from build123d import *

# Parameters (mm, degrees)
SKETCH1_R           = 1.79994
SKETCH1_R_2         = 1.5
BOSS_EXTRUDE1_DEPTH = 7
SKETCH2_W           = 75
SKETCH2_H           = 13.099999962
SKETCH2_R           = 2.6999438
SKETCH2_R_2         = 2.499995
SKETCH2_R_3         = 1.3498449
BOSS_EXTRUDE2_DEPTH = 6.987999994
SKETCH2_3_R         = 2.6999438
SKETCH2_3_R_2       = 1.3498449
CUT_EXTRUDE1_DEPTH  = 2.5
SKETCH7_W           = 45.754771374
SKETCH7_H           = 7.378762064
SKETCH7_W_2         = 5.75825354
SKETCH7_H_2         = 4.98011117
BOSS_EXTRUDE4_DEPTH = 7
SKETCH8_W           = 15.938133918
SKETCH8_H           = 10.613167284
CUT_EXTRUDE3_DEPTH  = 21.288
FILLET3_R           = 3.048
SKETCH4_W           = 25
SKETCH4_H           = 15.064836289
CUT_EXTRUDE2_DEPTH  = 38.822


with BuildPart() as part:
    # Sketch1 → Boss-Extrude1 (new body)
    with BuildSketch(Plane.XY):
        with BuildLine():
            Line((37.5, -10.5), (30, -10.5))
            ThreePointArc((30, -10.5), (25, -15.5), (20, -10.5))
            Line((20, -10.5), (5, -10.5))
            ThreePointArc((5, -10.5), (0, -15.5), (-5, -10.5))
            Line((-5, -10.5), (-20, -10.5))
            ThreePointArc((-20, -10.5), (-25, -15.5), (-30, -10.5))
            Line((-30, -10.5), (-37.5, -10.5))
            Line((-37.5, -10.5), (-37.5, 10.5))
            Line((-37.5, 10.5), (37.5, 10.5))
            Line((37.5, 10.5), (37.5, -10.5))
        make_face()
        with Locations((-25, -10.5)):
            Circle(SKETCH1_R, mode=Mode.SUBTRACT)
        with Locations((0, -10.5)):
            Circle(SKETCH1_R, mode=Mode.SUBTRACT)
        with Locations((25, -10.5)):
            Circle(SKETCH1_R, mode=Mode.SUBTRACT)
        with Locations((-35, 8)):
            Circle(SKETCH1_R_2, mode=Mode.SUBTRACT)
        with Locations((-15, 8)):
            Circle(SKETCH1_R_2, mode=Mode.SUBTRACT)
        with Locations((-10, 8)):
            Circle(SKETCH1_R_2, mode=Mode.SUBTRACT)
        with Locations((10, 8)):
            Circle(SKETCH1_R_2, mode=Mode.SUBTRACT)
        with Locations((35, 8)):
            Circle(SKETCH1_R_2, mode=Mode.SUBTRACT)
        with Locations((15, 8)):
            Circle(SKETCH1_R_2, mode=Mode.SUBTRACT)
    extrude(amount=BOSS_EXTRUDE1_DEPTH)

    # Sketch2 → Boss-Extrude2 (add)
    with BuildSketch(Plane(origin=(0, 2.24999999, 0), x_dir=(1, 0, 0), z_dir=(0, 1, 0))):
        with Locations((0, -13.549999981)):
            Rectangle(SKETCH2_W, SKETCH2_H)
        with Locations((31.0001404, -13.549999981)):
            Circle(SKETCH2_R, mode=Mode.SUBTRACT)
        with Locations((-31.0001404, -13.549999981)):
            Circle(SKETCH2_R, mode=Mode.SUBTRACT)
        with Locations((-25, -13.549999981)):
            Circle(SKETCH2_R_2, mode=Mode.SUBTRACT)
        with Locations((-6.0001404, -13.549999981)):
            Circle(SKETCH2_R, mode=Mode.SUBTRACT)
        with Locations((6.0001404, -13.549999981)):
            Circle(SKETCH2_R, mode=Mode.SUBTRACT)
        with Locations((0, -13.549999981)):
            Circle(SKETCH2_R_2, mode=Mode.SUBTRACT)
        with Locations((-18.9998596, -13.549999981)):
            Circle(SKETCH2_R, mode=Mode.SUBTRACT)
        with Locations((25, -13.549999981)):
            Circle(SKETCH2_R_2, mode=Mode.SUBTRACT)
        with Locations((18.9998596, -13.549999981)):
            Circle(SKETCH2_R, mode=Mode.SUBTRACT)
        with Locations((-31.0001404, -13.549999981)):
            Circle(SKETCH2_R)
        with Locations((-31.0001404, -13.549999981)):
            Circle(SKETCH2_R_3, mode=Mode.SUBTRACT)
        with Locations((-18.9998596, -13.549999981)):
            Circle(SKETCH2_R)
        with Locations((-18.9998596, -13.549999981)):
            Circle(SKETCH2_R_3, mode=Mode.SUBTRACT)
        with Locations((-6.0001404, -13.549999981)):
            Circle(SKETCH2_R)
        with Locations((-6.0001404, -13.549999981)):
            Circle(SKETCH2_R_3, mode=Mode.SUBTRACT)
        with Locations((6.0001404, -13.549999981)):
            Circle(SKETCH2_R)
        with Locations((6.0001404, -13.549999981)):
            Circle(SKETCH2_R_3, mode=Mode.SUBTRACT)
        with Locations((18.9998596, -13.549999981)):
            Circle(SKETCH2_R)
        with Locations((18.9998596, -13.549999981)):
            Circle(SKETCH2_R_3, mode=Mode.SUBTRACT)
        with Locations((31.0001404, -13.549999981)):
            Circle(SKETCH2_R)
        with Locations((31.0001404, -13.549999981)):
            Circle(SKETCH2_R_3, mode=Mode.SUBTRACT)
    extrude(amount=-BOSS_EXTRUDE2_DEPTH)

    # Sketch2<3> → Cut-Extrude1 (cut)
    with BuildSketch(Plane(origin=(0, 2.24999999, 0), x_dir=(1, 0, 0), z_dir=(0, 1, 0))):
        with Locations((-31.0001404, -13.549999981)):
            Circle(SKETCH2_3_R)
        with Locations((-31.0001404, -13.549999981)):
            Circle(SKETCH2_3_R_2, mode=Mode.SUBTRACT)
        with Locations((-18.9998596, -13.549999981)):
            Circle(SKETCH2_3_R)
        with Locations((-18.9998596, -13.549999981)):
            Circle(SKETCH2_3_R_2, mode=Mode.SUBTRACT)
        with Locations((-6.0001404, -13.549999981)):
            Circle(SKETCH2_3_R)
        with Locations((-6.0001404, -13.549999981)):
            Circle(SKETCH2_3_R_2, mode=Mode.SUBTRACT)
        with Locations((6.0001404, -13.549999981)):
            Circle(SKETCH2_3_R)
        with Locations((6.0001404, -13.549999981)):
            Circle(SKETCH2_3_R_2, mode=Mode.SUBTRACT)
        with Locations((18.9998596, -13.549999981)):
            Circle(SKETCH2_3_R)
        with Locations((18.9998596, -13.549999981)):
            Circle(SKETCH2_3_R_2, mode=Mode.SUBTRACT)
        with Locations((31.0001404, -13.549999981)):
            Circle(SKETCH2_3_R)
        with Locations((31.0001404, -13.549999981)):
            Circle(SKETCH2_3_R_2, mode=Mode.SUBTRACT)
    extrude(amount=-CUT_EXTRUDE1_DEPTH, mode=Mode.SUBTRACT)

    # Sketch7 → Boss-Extrude4 (add)
    with BuildSketch(Plane(origin=(0, 0, 0), x_dir=(-1, 0, 0), z_dir=(0, 0, -1))):
        with Locations((-0.544699659, 6.810618968)):
            Rectangle(SKETCH7_W, SKETCH7_H)
        with Locations((-0.155628474, -10.184996596)):
            Rectangle(SKETCH7_W_2, SKETCH7_H_2)
    extrude(amount=-BOSS_EXTRUDE4_DEPTH)

    # Sketch8 → Cut-Extrude3 (cut)
    with BuildSketch(Plane.XY.offset(7)):
        with Locations((2.969066959, -15.806583642)):
            Rectangle(SKETCH8_W, SKETCH8_H)
    extrude(amount=-CUT_EXTRUDE3_DEPTH, mode=Mode.SUBTRACT)

    # Fillet3
    fillet3_edges = [part.edges().sort_by_distance(p)[0] for p in [
        (-37.5, 10.5, 3.5),
        (37.5, 10.5, 3.5),
        (37.5, -10.5, 3.5),
        (-37.5, -10.5, 3.5),
        (37.5, -1.244000007, 20.099999962),
        (-37.5, -1.244000007, 20.099999962),
    ]]
    fillet(fillet3_edges, radius=FILLET3_R)

    # Sketch4 → Cut-Extrude2 (cut)
    with BuildSketch(Plane.XY.offset(7)):
        with Locations((0, -12.270418149)):
            Rectangle(SKETCH4_W, SKETCH4_H)
    extrude(amount=-CUT_EXTRUDE2_DEPTH, mode=Mode.SUBTRACT)


solid = part.part
Can you work these out from the model? Positions are in its coordinate system, mm. A direction names the side the tool comes from. Coordinates: 2 decimals unless noted, no trailing zeros. Order: outer loops, then holes, each group sorted by start corner. A loop starts at its lowest first (then second) coordinate and runs counter-clockwise, first axis right, second up. Notation, with made-up numbers: M -16,11.25 L 30,11.25 A21 cw 30,24.25 Z; hole C 60.25,12.5 d8. An arc over 180 degrees is marked long. Answer as CSV lines item,"result".
(1) Suppose I cut it at A-A on z = 5.5. Please give me the cut outline in (x, y), plus the area to 3 significant figures.
Geometry check:
outline,"M -37.5,-7.45 A3.05 ccw -34.45,-10.5 L -30,-10.5 A5 ccw -20,-10.5 L -12.5,-10.5 L -12.5,-4.74 L 12.5,-4.74 L 12.5,-10.5 L 20,-10.5 A5 ccw 30,-10.5 L 34.45,-10.5 A3.05 ccw 37.5,-7.45 L 37.5,7.45 A3.05 ccw 34.45,10.5 L -34.45,10.5 A3.05 ccw -37.5,7.45 Z; hole C -35,8 d3; hole C -25,-10.5 d3.6; hole C 25,-10.5 d3.6; hole C 35,8 d3"
area,"1,470 mm^2"
(2) Suppose I cut it at C-C on y = -1.25. Count the separate pieces of the cut face and the enclosed holes in it, plus the area to 3 significant figures.
Geometry check:
separate pieces,"1"
enclosed holes,"9"
area,"1,410 mm^2"
(3) Suppose I cut it at B-B on x = -25. Please give me the cut outline in (y, z), plus the area to 3 significant figures.
Geometry check:
outline,"M -15.5,0 L -12.3,0 L -12.3,7 L -15.5,7 Z; M -8.7,0 L 10.5,0 L 10.5,7 L 2.25,7 L 2.25,11.05 L -4.74,11.05 L -4.74,7 L -8.7,7 Z; M -4.74,16.05 L 2.25,16.05 L 2.25,20.1 L -4.74,20.1 Z"
area,"213 mm^2"
(4) On a 3-axis mill with a long thin cutter (end or side, diameter ignored), from which of +Z, -Z, +X, -X, +Y, -Y can I reach the whole of each face in a straight line? I mean faces 5 (the flat face through (-18, -0.25, 12)), 6 (the flat face through (-12.5, -8, 4)), 7 (the flat face through (-1, 2.25, 11)), 8 (the flat face through (-32, -10.5, 3)). Say none if no direction works.
Geometry check:
face 5,"+Y"
face 6,"+Z, -Z, -Y"
face 7,"+Z, +X, -X, +Y"
face 8,"+Z, -Z, -X, -Y"
(5) Suppose I cut it at D-D on x = -0.5. Please give me the cut outline in (y, z).
Geometry check:
outline,"M -4.74,0 L 10.5,0 L 10.5,7 L 2.25,7 L 2.25,11.1 L -4.74,11.1 Z; M -4.74,16 L 2.25,16 L 2.25,20.1 L -4.74,20.1 Z"
(6) Please list where these lines run through material, in increasing order: L1, parallel to Z at x = 18, y = 3; L2, parallel to Y at x = 25, z = 2.75; L3, parallel to X at y = 6.75, z = 4.5.
Geometry check:
L1,"0 to 7"
L2,"-15.5 to -12.3, -8.7 to 10.5"
L3,"-37.5 to -35.83, -34.17 to 34.17, 35.83 to 37.5"
(7) I'm going to push flat-ended pins straight in: pin 1 (5.5 mm diameter, centred on x = 25, y = -8.5, fed in from +Z); pin 2 (4.5 mm diameter, centred on x = 6, z = 13.55, fed in from -Y); pin 3 (8 mm diameter, centred on x = -25, z = 13.55, fed in from +Y); pin 4 (5 mm diameter, centred on x = -35, y = 8, fed in from -Z). Where does each tip first touch, or does it pass through?
Geometry check:
pin 1,"z = 7"
pin 2,"y = -4.74"
pin 3,"y = 2.25"
pin 4,"z = 0"
(8) If we mould it in two halves opening along Z, with no side actions, what happens to faces 1 (the flat face through (37.5, 0, 7)), 2 (the flat face through (1, 1, 0)), 3 (the flat face through (32, -0.25, 12)), 4 (the cylindrical face through (-28.506, 1.017, 14.584))? For each: released by +Z, released by -Z, zero draft, split by the parting line, or undercut.
Geometry check:
face 1,"zero draft"
face 2,"released by -Z"
face 3,"undercut"
face 4,"undercut"
